Autodesk Inventor part; units mm, degrees
ref_plane "YZ Plane" through (0, 0, 0) normal (1, 0, 0) x (0, 1, 0)
ref_plane "XZ Plane" through (0, 0, 0) normal (0, 1, 0) x (-1, 0, 0)
ref_plane "XY Plane" through (0, 0, 0) normal (0, 0, 1) x (1, 0, 0)
sketch "草图1" plane through (0, 0, 0) normal (0, 0, 1) x (1, 0, 0)
  line L0 (10, -22.5) -> (-10, -22.5)
  line L1 (-10, -22.5) -> (-10, 22.5)
  line L2 (-10, 22.5) -> (10, 22.5)
  line L3 (10, 22.5) -> (10, -22.5)
  line L4 (10, -22.5) -> (-10, 22.5) construction
  line L5 (-10, -22.5) -> (10, 22.5) construction
  line L6 (9, 21.5) -> (-9, 21.5)
  line L7 (-9, 21.5) -> (-9, -21.5)
  line L8 (-9, -21.5) -> (9, -21.5)
  line L9 (9, -21.5) -> (9, 21.5)
  point P0 (0, 0)
  dimension "d0" = 45
  dimension "d1" = 20
  dimension "d4" = 1
extrude "拉伸1" add sketch "草图1" along normal blind 328
sketch "草图4" plane through (-10, 22.5, 0) normal (0, 1, 0) x (1, 0, 0)
  circle A0 centre (9, -81) radius 2
  circle A1 centre (9, -97) radius 2
  line L0 (0, 0) -> (0, -328)
  line L1 (20, 0) -> (0, 0)
  line L2 (0, -164) -> (-22.908, -164)
  circle A2 centre (9, -247) radius 2
  circle A3 centre (9, -231) radius 2
  point P0 (10, 0)
  dimension "d5" = 9
  dimension "d6" = 16
  dimension "d7" = 81
extrude "拉伸2" cut sketch "草图4" against normal blind 58.75
sketch "草图5" plane through (0, 0, 328) normal (0, 0, 1) x (1, 0, 0)
  line L0 (10, 22.5) -> (-10, 22.5)
  line L1 (-10, 22.5) -> (-10, -22.5)
  line L2 (-10, -22.5) -> (10, -22.5)
  line L3 (10, -22.5) -> (10, 22.5)
  line L4 (9, 21.5) -> (9, -21.5)
  line L5 (9, -21.5) -> (-9, -21.5)
  line L6 (-9, -21.5) -> (-9, 21.5)
  line L7 (-9, 21.5) -> (9, 21.5)
  point P0 (0, 0)
ref_plane "工作平面1" through (0, 0, 164) normal (0, 0, 1) x (1, 0, 0)
extrude "拉伸3" add sketch "草图5" along normal blind 50
mirror "镜像1" about plane through (0, 0, 164) normal (0, 0, 1) of "拉伸3"
properties part number "321x30"
Work out the finished part from the listing and answer in its coordinate system (mm). A direction names the side the tool comes from. Coordinates: 2 decimals unless noted, no trailing zeros. Loops run counter-clockwise (first coordinate to the right, second up) from the corner with the lowest first, then second, coordinate; pieces in that order, holes last. Notation, with made-up numbers: M 23,43.5 L 76,43.5 A14 cw 76,50.5 Z; hole C -19.5,-29.5 d6. An arc over 180 degrees is marked long. Answer in a Markdown table with one row per item. Add a question column.
1. Find section B-B, the plane z = 305.5. Write down the section's boundary in (x, y).
2. The mould has two halves that part along Y. Classify faces 1 (the flat face through (9, 0, 167)), 2 (the flat face through (0, -22.5, 167)), 3 (the flat face through (10, 0, 167)): pulls with the +Y half, pulls with the -Y half, needs draft (parallel to the pull), parting line crosses it, or undercut.
3. A flat-ended cylindrical pin translates along its axis: P1, Ø4.5, axis at x = -1, z = 81, coming from the -Y side. Find the tip coordinate at first contact, or state that the pin passes through.
4. Consider L1, parallel to Z at x = -1, y = 21.7; L2, parallel to X at y = -22, z = 81; L3, parallel to X at y = 7.5, z = 38. Determine where each line is inside the solid, lowest interval first.
5. A tool of negligible diameter and unlimited length cuts with its end or side. For faces 4 (the flat face through (0, -21.5, 167)), 5 (the flat face through (0, 22.5, 167)), from which of +Z, -Z, +X, -X, +Y, -Y can it reach the whole face along a straight path? Write none if from no direction.
6. Find section A-A, the plane y = -7. Write down the section's boundary in (x, z), then the cut area to 3 significant figures.
Reported:
| question | item | result |
|---|---|---|
| 1 | outline | M -10,-22.5 L 10,-22.5 L 10,22.5 L -10,22.5 Z; hole M -9,-21.5 L 9,-21.5 L 9,21.5 L -9,21.5 Z |
| 2 | face 1 | undercut |
| 2 | face 2 | pulls with the -Y half |
| 2 | face 3 | needs draft |
| 3 | P1 | stops at y = -22.5 |
| 4 | L1 | z = -50 to 79, 83 to 95, 99 to 229, 233 to 245, 249 to 378 |
| 4 | L2 | x = -10 to -3, 1 to 10 |
| 4 | L3 | x = -10 to -9, 9 to 10 |
| 5 | face 4 | +Z, -Z |
| 5 | face 5 | +Z, -Z, +X, -X, +Y |
| 6 | outline | M -10,-50 L -9,-50 L -9,378 L -10,378 Z; M 9,-50 L 10,-50 L 10,378 L 9,378 Z |
| 6 | area | 856 mm^2 |
